The model under review builds one solid part; all positions refer to its coordinate system, in mm. Give positions to 0.01 mm unless a question says otherwise; leave off trailing zeros. Write each loop counter-clockwise with the first axis right and the second up, starting at its lowest first coordinate (ties: lowest second). Pieces come first, ordered by that corner, then holes. Notation, with made-up numbers: M -29,23.5 L -5,23.5 A36 ccw -5,62.5 Z; hole C 40.25,63.25 d1. An arc over 180 degrees is marked long. Write item = value, one per line. Start each with the question number.
Autodesk Inventor part; units mm, degrees
ref_plane "YZ Plane" through (0, 0, 0) normal (1, 0, 0) x (0, 1, 0)
ref_plane "XZ Plane" through (0, 0, 0) normal (0, 1, 0) x (-1, 0, 0)
ref_plane "XY Plane" through (0, 0, 0) normal (0, 0, 1) x (1, 0, 0)
sketch "Sketch1" plane through (0, 0, 0) normal (0, 0, 1) x (1, 0, 0)
  line L0 (47.6451, -34.29) -> (92.334, -34.29)
  line L1 (47.6451, -34.29) -> (41.1035, -34.29)
  line L2 (39.8575, 12.7612) -> (31.599, 12.7612)
  line L3 (39.8575, 12.7612) -> (20.8075, 12.7612)
  line L4 (79.512, 12.7612) -> (37.4294, 12.7612)
  line L5 (79.512, -31.9773) -> (79.512, 12.7612)
  line L6 (92.334, -18.8499) -> (92.334, 1.5256)
  line L7 (92.334, -18.8499) -> (92.334, -34.29)
  circle A0 centre (85.7451, -25.4) radius 3.9624
  circle A1 centre (85.7451, -12.7) radius 2.1844
  circle A2 centre (73.0451, -12.7) radius 2.54
  circle A3 centre (60.3451, -12.7) radius 2.54
  circle A4 centre (73.0451, -25.4) radius 2.54
  line L8 (-341.1851, -3.2325) -> (91.1147, -3.2325)
  line L9 (25.7365, 2.0147) -> (20.8075, 12.7612)
  line L10 (91.1147, -3.2325) -> (92.334, -3.2325)
  circle A5 centre (85.7451, -25.4) radius 5.08
  line L11 (39.8575, 12.7612) -> (8.1075, 12.7612)
  line L12 (8.1075, 12.7612) -> (56.4583, -56.2272)
  line L13 (41.1035, -35.5589) -> (41.9728, -35.5589)
  line L14 (41.9728, -35.5589) -> (92.334, -35.5589)
  line L15 (92.334, -35.5589) -> (92.334, -34.29)
  point P0 (0, 0)
  point P1 (0, 0)
  point P2 (41.3274, -31.9773)
  point P3 (79.512, -18.8499)
  point P4 (79.512, -3.2325)
  point P5 (79.512, -3.2325)
  dimension "d0" = 19.05
  dimension "d1" = 432.2999
  dimension "d2" = 10.16
  dimension "d3" = 31.75
extrude "Extrusion1" add sketch "Sketch1" along normal blind 1.5875 contours L4 L5 L8 L12 L11 L3 L2 | L8 L10 L6 L7 L15 L14 L12
fillet "Fillet1" radius 6.35 5 edges at (79.512, 12.7612, 0.7937) (79.512, -3.2325, 0.7937) (92.334, -3.2325, 0.7937) (92.334, -35.5589, 0.7937) (41.9728, -35.5589, 0.7937)
fillet "Fillet2" radius 3.175 1 edges at (8.1075, 12.7612, 0.7937)
properties part number "Sleds poly V4"
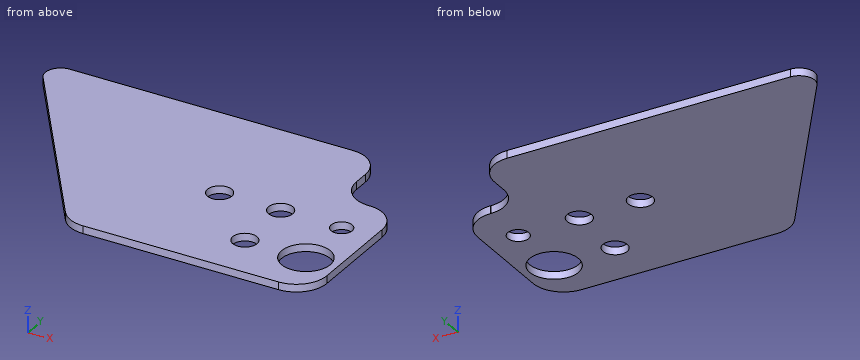
Item 1: Clearance check with flat-ended pins moving along their axes: P1, Ø4.5, axis at x = 60.35, y = -12.7, coming from the +Z side; P2, Ø0.8, axis at y = 4.5, z = 0.5, coming from the +X side. State where each tip first meets the part, or that it passes through.
Item 2: To check wall thickness, follow probe 1 along X at (y, z) = (-27, 0.85); probe 2 along X at (y, z) = (-12.5, 1.4); probe 3 along Y at (x, z) = (58.5, 0.35). State the ranges of each line that lie inside material, in increasing order. Write a range as [from, to].
Item 3: We need section A-A, the plane z = 1.3. Give the number of separate pieces and of enclosed holes in the cut face, and give its area (3 significant figures).
Item 4: We need section B-B, the plane y = -25.4. Write out the cut boundary in (x, z).
Item 5: We need section C-C, the plane y = -12.7. Write out the cut boundary in (x, z).
Item 6: We need section D-D, the plane x = 23. Write out the cut boundary in (y, z).
Worked out:
q1.P1 = through
q1.P2 = 79.51
q2.probe_1 = [35.97, 71.07], [75.02, 80.92], [90.57, 92.33]
q2.probe_2 = [25.81, 57.81], [62.88, 70.51], [75.58, 83.57], [87.92, 92.33]
q2.probe_3 = [-35.56, -14.45], [-10.95, 12.76]
q3.separate_pieces = 1
q3.enclosed_holes = 5
q3.area = 2,860 mm²
q4.outline = M 34.85,0 L 70.51,0 L 70.51,1.59 L 34.85,1.59 Z; M 75.59,0 L 80.67,0 L 80.67,1.59 L 75.59,1.59 Z; M 90.83,0 L 92.33,0 L 92.33,1.59 L 90.83,1.59 Z
q5.outline = M 25.95,0 L 57.81,0 L 57.81,1.59 L 25.95,1.59 Z; M 62.89,0 L 70.51,0 L 70.51,1.59 L 62.89,1.59 Z; M 75.59,0 L 83.56,0 L 83.56,1.59 L 75.59,1.59 Z; M 87.93,0 L 92.33,0 L 92.33,1.59 L 87.93,1.59 Z
q6.outline = M -8.49,0 L 12.76,0 L 12.76,1.59 L -8.49,1.59 Z
